Can you work these out from the drawing? Everything is in mm from the part's minimum corner. Give positions to 0.01 mm unless a question says otherwise; leave off trailing zeros. Write each loop counter-clockwise with the first axis right and the second up, starting at its lowest first coordinate (ties: lowest second). Pieces come first, ordered by that corner, then holes. Notation, with made-up numbers: (51, 80.25) - (92, 80.25) arc R19 ccw to (92, 115.25) - close; hole circle Ø8 at (29, 66). An arc over 180 degrees is marked (long way). Answer in a Markdown table with one row per item.
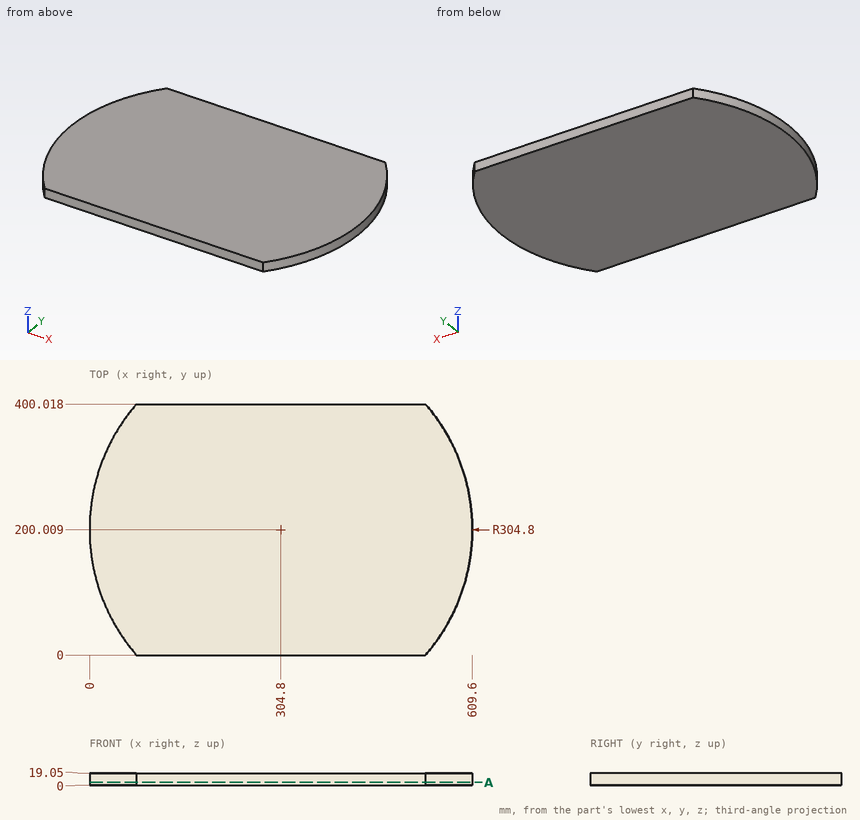
1) Will these pins go through, and if not, where does the flat tip stop? P1, Ø3, axis at y = 204.5, z = 13.5, coming from the +X side (1 decimal); P2, Ø4, axis at y = 323, z = 14, coming from the -X side; P3, Ø2, axis at y = 98.5, z = 12.5, coming from the -X side.
Check values:
| item | result |
|---|---|
| P1 | stops at x = 609.6 |
| P2 | stops at x = 25.04 |
| P3 | stops at x = 17.05 |
2) If I drill on line 1 (Y direction, x = 539, z = 15.5) (1 decimal); line 2 (X direction, y = 115.5, z = 15.75); line 3 (X direction, y = 36, z = 3), over which ranges is the centre line in solid material (lowest first)?
Check values:
| item | result |
|---|---|
| line 1 | y = 4.9 to 395.1 |
| line 2 | x = 11.95 to 597.65 |
| line 3 | x = 47.89 to 561.71 |
3) Imagine slicing it at A-A (z = 4.25). List the corners of the cut face in (x, y) for me, then the cut area to 3 significant figures.
Check values:
| item | result |
|---|---|
| outline | (74.8, 0) - (534.8, 0) arc R304.8 ccw to (534.8, 400.02) - (74.8, 400.02) arc R304.8 ccw to start |
| area | 225,000 mm2 |
